Could you check a few things on this model? Use its own coordinates, in mm. A direction names the side the tool comes from. Give positions to 0.01 mm unless a question says otherwise; leave off trailing zeros. Loops run counter-clockwise (first coordinate to the right, second up) from the corner with the lowest first, then second, coordinate; pieces in that order, holes last. Notation, with made-up numbers: M -25.75,42.5 L 15.25,42.5 A12 ccw 15.25,62.5 Z; hole C 1,87 d2. An arc over 180 degrees is marked long. Answer in a Markdown table with one row per item. Add a question column.
1. If we section it at C-C on y = 4: List the corners of the cut face in (x, z) for me.
2. I need wall thicknesses on line 1 along X through (y, z) = (71, 12.5); line 2 along Y through (x, z) = (17.5, 6.5); line 3 along Y through (x, z) = (34.05, 10). Which ranges of each line are inside material? Lowest first, please. Write a range as from..to.
3. If we section it at D-D on z = 10: Count the separate pieces of the cut face and the enclosed holes in it, then the cut area to 3 significant figures.
4. Thinking about a two-plate mould opening in X: for faces 6 (the flat face through (26.771, 5.317, 9.86)), 7 (the flat face through (30.208, 1.683, 9.86)), 8 (the cylindrical face through (34.003, 64.804, 9.738)), which applies, released by +X, released by -X, zero draft, split by the parting line, or undercut?
5. Which directions (+Z, -Z, +X, -X, +Y, -Y) give clear straight access to the entire face, cutting with the end or side of a thin tool? Please do faces 1 (the flat face through (18, -1, 10)), 2 (the flat face through (34.51, 40, 1)), 3 (the cylindrical face through (-32.045, 75.983, 10.22)), 4 (the cylindrical face through (32.045, 10.987, 9.846)), 5 (the flat face through (-33.51, 66, 10)).
6. If we section it at B-B on x = 0: List the corners of the cut face in (y, z) for me (3 decimals).
7. If we section it at A-A on y = 32: List the corners of the cut face in (x, z) for me, then the cut area to 3 significant figures.
8. I'm going to push flat-ended pins straight in: pin 1 Ø1 at (x, z) = (21.5, 9) entering from +Y; pin 2 Ø6 at (x, z) = (12, 10.5) entering from -Y; pin 3 Ø2 at (x, z) = (0, 10) entering from -Y; pin 4 Ø5 at (x, z) = (-24, 9) entering from +Y. Where does each tip first touch, or does it pass through?
```python
from build123d import *

# Parameters (mm, degrees)
BOSS_EXTRUDE1_DEPTH = 20
FILLET2_RADIUS      = 10
FILLET2_LENGTH      = 5
FILLET3_RADIUS      = 10
FILLET3_LENGTH      = 5
SKETCH2_W           = 36
SKETCH2_H           = 7.55
CUT_EXTRUDE1_DEPTH  = 3
CUT_EXTRUDE2_REACH  = 87.375
SKETCH4_R           = 1.21
SKETCH6_W           = 10
SKETCH6_H           = 7.55
CUT_EXTRUDE3_DEPTH  = 1
SKETCH7_R           = 2.45
CUT_EXTRUDE4_DEPTH  = 4
CUT_EXTRUDE5_REACH  = 105.925
SKETCH9_R           = 1.21
SKETCH10_R          = 2.475
CUT_EXTRUDE6_DEPTH  = 4
CUT_EXTRUDE7_DEPTH  = 105.582615121


with BuildPart() as part:
    # Sketch1 → Boss-Extrude1 (new body)
    with BuildSketch(Plane.XY):
        Polygon((-26.024718626, -2.5), (26.024718626, -2.5), (34.51, 5.985281374), (34.51, 75.985281374), (29.51, 75.985281374), (29.51, 8.056349186), (23.953650814, 2.5), (-23.953650814, 2.5), (-29.51, 8.056349186), (-29.51, 75.985281374), (-34.51, 75.985281374), (-34.51, 5.985281374), align=None)
    extrude(amount=BOSS_EXTRUDE1_DEPTH)

    # Fillet2: full round fillet: the end face becomes a half cylinder, R = half its width
    fillet2_face = Plane((-32.01, 75.985281374, 10), x_dir=(-1, 0, 0), z_dir=(0, 1, 0))  # on the end face: x along it, z out of the body
    fillet2_slab = fillet2_face.offset(-FILLET2_RADIUS / 2) * Box(FILLET2_LENGTH, 2 * FILLET2_RADIUS, FILLET2_RADIUS, mode=Mode.PRIVATE)  # the body's end, R deep
    fillet2_round = Plane((-32.01, 65.985281374, 10), x_dir=(0, 1, 0), z_dir=(-1, 0, 0)) * Cylinder(FILLET2_RADIUS, FILLET2_LENGTH, mode=Mode.PRIVATE)  # its axis R under the face
    add(fillet2_slab - fillet2_round, mode=Mode.SUBTRACT)

    # Fillet3: full round fillet: the end face becomes a half cylinder, R = half its width
    fillet3_face = Plane((32.01, 75.985281374, 10), x_dir=(1, 0, 0), z_dir=(0, 1, 0))  # on the end face: x along it, z out of the body
    fillet3_slab = fillet3_face.offset(-FILLET3_RADIUS / 2) * Box(FILLET3_LENGTH, 2 * FILLET3_RADIUS, FILLET3_RADIUS, mode=Mode.PRIVATE)  # the body's end, R deep
    fillet3_round = Plane((32.01, 65.985281374, 10), x_dir=(0, 1, 0), z_dir=(1, 0, 0)) * Cylinder(FILLET3_RADIUS, FILLET3_LENGTH, mode=Mode.PRIVATE)  # its axis R under the face
    add(fillet3_slab - fillet3_round, mode=Mode.SUBTRACT)

    # Sketch2 → Cut-Extrude1 (cut)
    with BuildSketch(Plane.XZ.offset(2.5)):
        with Locations((0, 10)):
            Rectangle(SKETCH2_W, SKETCH2_H)
    extrude(amount=-CUT_EXTRUDE1_DEPTH, mode=Mode.SUBTRACT)

    # Sketch4 → Cut-Extrude2 (cut, up to next)
    with BuildSketch(Plane.XZ.offset(-0.5), mode=Mode.PRIVATE) as cut_extrude2_sk1:
        with Locations(Location((0, 10, 0), (0, 0, 270))):
            Circle(SKETCH4_R)
    cut_extrude2_tool1 = extrude(cut_extrude2_sk1.sketch, amount=-CUT_EXTRUDE2_REACH, mode=Mode.PRIVATE) & part.part
    add(cut_extrude2_tool1.solids().sort_by_distance((0, 0.5, 10))[0], mode=Mode.SUBTRACT)

    # Sketch6 → Cut-Extrude3 (cut)
    with BuildSketch(Plane.XZ.offset(-0.5)):
        with Locations((0, 10)):
            Rectangle(SKETCH6_W, SKETCH6_H)
    extrude(amount=-CUT_EXTRUDE3_DEPTH, mode=Mode.SUBTRACT)

    # Sketch7 → Cut-Extrude4 (cut)
    with BuildSketch(Plane.ZY.offset(-29.51)):
        with Locations(Location((10, 65.985281374, 0), (0, 0, 270))):
            Circle(SKETCH7_R)
    extrude(amount=-CUT_EXTRUDE4_DEPTH, mode=Mode.SUBTRACT)

    # Sketch9 → Cut-Extrude5 (cut, up to next)
    with BuildSketch(Plane.ZY.offset(-33.51), mode=Mode.PRIVATE) as cut_extrude5_sk1:
        with Locations((10, 65.985281374)):
            Circle(SKETCH9_R)
    cut_extrude5_tool1 = extrude(cut_extrude5_sk1.sketch, amount=-CUT_EXTRUDE5_REACH, mode=Mode.PRIVATE) & part.part
    add(cut_extrude5_tool1.solids().sort_by_distance((33.51, 65.985281, 10))[0], mode=Mode.SUBTRACT)

    # Sketch10 → Cut-Extrude6 (cut)
    with BuildSketch(Plane(origin=(-29.51, 0, 0), x_dir=(0, 0, -1), z_dir=(1, 0, 0))):
        with Locations(Location((-10, 65.985281374, 0), (0, 0, 90))):
            Circle(SKETCH10_R)
    extrude(amount=-CUT_EXTRUDE6_DEPTH, mode=Mode.SUBTRACT)

    # Sketch11 → Cut-Extrude7 (cut, through all)
    with BuildSketch(Plane(origin=(34.51, 0, 0), x_dir=(0, 0, -1), z_dir=(1, 0, 0))):
        with BuildLine():
            Line((-3, 53.985281374), (-3, 17.985281374))
            ThreePointArc((-3, 17.985281374), (-10, 10.985281374), (-17, 17.985281374))
            Line((-17, 17.985281374), (-17, 53.985281374))
            ThreePointArc((-17, 53.985281374), (-10, 60.985281374), (-3, 53.985281374))
        make_face()
    extrude(amount=-CUT_EXTRUDE7_DEPTH, mode=Mode.SUBTRACT)


solid = part.part
```
Results:
| question | item | result |
|---|---|---|
| 1 | outline | M -32.52,0 L -25.45,0 L -25.45,20 L -32.52,20 Z; M 25.45,0 L 32.52,0 L 32.52,20 L 25.45,20 Z |
| 2 | line 1 | -34.51..-29.51, 29.51..34.51 |
| 2 | line 2 | 0.5..2.5 |
| 2 | line 3 | 5.53..10.99, 60.99..64.78, 67.2..75.99 |
| 3 | separate pieces | 5 |
| 3 | enclosed holes | 0 |
| 3 | area | 377 mm2 |
| 4 | face 6 | undercut |
| 4 | face 7 | released by +X |
| 4 | face 8 | zero draft |
| 5 | face 1 | -Y |
| 5 | face 2 | +Z, -Z, +X, +Y, -Y |
| 5 | face 3 | +X, -X, +Y |
| 5 | face 4 | +X, -X |
| 5 | face 5 | none |
| 6 | outline | M -2.5,0 L 2.5,0 L 2.5,8.79 L 1.5,8.79 L 1.5,6.225 L -2.5,6.225 Z; M -2.5,13.775 L 1.5,13.775 L 1.5,11.21 L 2.5,11.21 L 2.5,20 L -2.5,20 Z |
| 7 | outline | M -34.51,0 L -29.51,0 L -29.51,3 L -34.51,3 Z; M -34.51,17 L -29.51,17 L -29.51,20 L -34.51,20 Z; M 29.51,0 L 34.51,0 L 34.51,3 L 29.51,3 Z; M 29.51,17 L 34.51,17 L 34.51,20 L 29.51,20 Z |
| 7 | area | 60.0 mm2 |
| 8 | pin 1 | y = 2.5 |
| 8 | pin 2 | y = 0.5 |
| 8 | pin 3 | through |
| 8 | pin 4 | y = 5.05 |
